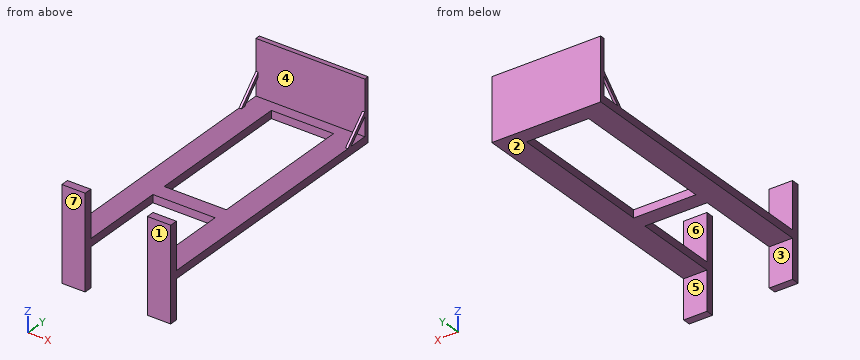
```python
from build123d import *

# Parameters (mm, degrees)
SALIENTE_EXTRUIR1_DEPTH        = 300
SALIENTE_EXTRUIR1_DEPTH_BACK   = 300
CROQUIS1_W                     = 150
CROQUIS1_H                     = 50
SALIENTE_EXTRUIR1_2_DEPTH      = 300
SALIENTE_EXTRUIR1_2_DEPTH_BACK = 300
CROQUIS2_W                     = 150
CROQUIS2_H                     = 50
SALIENTE_EXTRUIR2_DEPTH        = 1700
CROQUIS3_W                     = 700
CROQUIS3_H                     = 100
SALIENTE_EXTRUIR3_DEPTH        = 50
CROQUIS4_W                     = 700
CROQUIS4_H                     = 30
SALIENTE_EXTRUIR4_DEPTH        = 350
SALIENTE_EXTRUIR5_DEPTH        = 15
SALIENTE_EXTRUIR6_DEPTH        = 15


with BuildPart() as part:
    # Croquis1 → Saliente-Extruir1 (new, two sides: drawn at the far end of the back side and taken through both)
    with BuildSketch(Plane.XY.offset(-SALIENTE_EXTRUIR1_DEPTH_BACK)):
        with Locations((75, 25)):
            Rectangle(CROQUIS1_W, CROQUIS1_H)
    extrude(amount=SALIENTE_EXTRUIR1_DEPTH + SALIENTE_EXTRUIR1_DEPTH_BACK)



with BuildPart() as body_2:
    # Croquis1 → Saliente-Extruir1 2 (new, two sides: drawn at the far end of the back side and taken through both)
    with BuildSketch(Plane.XY.offset(-SALIENTE_EXTRUIR1_2_DEPTH_BACK)):
        with Locations((625, 25)):
            Rectangle(CROQUIS1_W, CROQUIS1_H)
    extrude(amount=SALIENTE_EXTRUIR1_2_DEPTH + SALIENTE_EXTRUIR1_2_DEPTH_BACK)


with BuildPart() as part_1:
    add(part.part)

    add(body_2.part)  # Saliente-Extruir2 merges body 2
    # Croquis2 → Saliente-Extruir2 (add)
    with BuildSketch(Plane(origin=(0, 50, 0), x_dir=(1, 0, 0), z_dir=(0, 1, 0))):
        with Locations((75, 25)):
            Rectangle(CROQUIS2_W, CROQUIS2_H)
        with Locations((625, 25)):
            Rectangle(CROQUIS2_W, CROQUIS2_H)
    extrude(amount=SALIENTE_EXTRUIR2_DEPTH)

    # Croquis3 → Saliente-Extruir3 (add)
    with BuildSketch(Plane.XY):
        with Locations((350, 650)):
            Rectangle(CROQUIS3_W, CROQUIS3_H)
        with Locations((350, 1700)):
            Rectangle(CROQUIS3_W, CROQUIS3_H)
    extrude(amount=-SALIENTE_EXTRUIR3_DEPTH)

    # Croquis4 → Saliente-Extruir4 (add)
    with BuildSketch(Plane.XY):
        with Locations((350, 1735)):
            Rectangle(CROQUIS4_W, CROQUIS4_H)
    extrude(amount=SALIENTE_EXTRUIR4_DEPTH)

    # Croquis5 → Saliente-Extruir5 (add)
    with BuildSketch(Plane.ZY):
        Polygon((0, 1570), (150, 1720), (120, 1720), (0, 1600), align=None)
    extrude(amount=-SALIENTE_EXTRUIR5_DEPTH)

    # Croquis6 → Saliente-Extruir6 (add)
    with BuildSketch(Plane(origin=(700, 0, 0), x_dir=(0, 0, -1), z_dir=(1, 0, 0))):
        Polygon((0, 1570), (0, 1600), (-120, 1720), (-150, 1720), align=None)
    extrude(amount=-SALIENTE_EXTRUIR6_DEPTH)


solid = part_1.part
```
Part model, mm, in its own coordinate system. Face numbers are marked on the shaded views. A direction names the side the tool comes from. Round coordinates to 2 decimals unless told otherwise and drop trailing zeros. Write each loop counter-clockwise with the first axis right and the second up, starting at its lowest first coordinate (ties: lowest second). Pieces come first, ordered by that corner, then holes.
Item 1: Cut at B-B, the plane x = 430.5. Give the cut face in (y, z).
Results:
outline: (600, -50) - (700, -50) - (700, 0) - (600, 0) - close; (1650, -50) - (1750, -50) - (1750, 350) - (1720, 350) - (1720, 0) - (1650, 0) - close
Item 2: Cut at C-C, the plane y = 1003. Give the cut face in (x, z).
Results:
outline: (0, -50) - (150, -50) - (150, 0) - (0, 0) - close; (550, -50) - (700, -50) - (700, 0) - (550, 0) - close
Item 3: Two-plate mould, pull along Y, no slides. Class the marked faces 1, 2, 3 and 4: +Y half, -Y half, draft (parallel to the pull), parting line (faces both ways), or undercut.
Results:
face 1: -Y half
face 2: draft
face 3: +Y half
face 4: undercut
Item 4: Cut at A-A, the plane z = 224. Give the cut face in (x, y).
Results:
outline: (0, 0) - (150, 0) - (150, 50) - (0, 50) - close; (0, 1720) - (700, 1720) - (700, 1750) - (0, 1750) - close; (550, 0) - (700, 0) - (700, 50) - (550, 50) - close
Item 5: Probe L1, parallel to X at y = 475.5, z = -27; L2, parallel to Y at x = 640, z = 284; L3, parallel to Y at x = 249.5, z = 182. List the from-to ranges inside material, lowest first.
Results:
L1: x = 0 to 150, 550 to 700
L2: y = 0 to 50, 1720 to 1750
L3: y = 1720 to 1750
Item 6: Cut at D-D, the plane z = -161. Give the cut face in (x, y), plus the area to 3 significant figures.
Results:
outline: (0, 0) - (150, 0) - (150, 50) - (0, 50) - close; (550, 0) - (700, 0) - (700, 50) - (550, 50) - close
area: 15,000 mm2
Item 7: Which spindle directions (+Z, -Z, +X, -X, +Y, -Y) get a long thin tool onto all of the face, cutting with end or side? Do the marked faces 5, 6 and 7. Say none if no direction does.
Results:
face 5: -Z, +X, -X, +Y
face 6: +Z, +X, -X
face 7: +Z, -Z, +X, -X, -Y
